Job drawing, mm, ordinate dimensions from the low corner. One solid piece. A direction names the side the tool comes from. Give positions to 0.01 mm unless a question says otherwise; leave off trailing zeros. Write each loop counter-clockwise with the first axis right and the second up, starting at its lowest first coordinate (ties: lowest second). Pieces come first, ordered by that corner, then holes. Notation, with made-up numbers: M -25,19.25 L 3,19.25 A24 ccw 3,30.25 Z; hole C 36.25,-38.5 d6. An arc over 180 degrees is marked long. Answer as CSV lines item,"result". Start each with the question number.
Item 1: Band-saw the part on C-C, the plane y = 2. List the corners of the cut face in (x, z) (1 decimal).
Item 2: Band-saw the part on A-A, the plane x = 31.3. List the corners of the cut face in (y, z).
Item 3: 3-axis set-ups, long thin cutter, end or side, ignore diameter. For the marked faces 4, 5, 6, 7 and 8: which of +Z, -Z, +X, -X, +Y, -Y reach the whole face in a straight line?
Item 4: Pin check, flat tips, straight feed: pin 1 (6 mm diameter, centred on y = 8.5, z = 21, fed in from +X); pin 2 (4 mm diameter, centred on x = 15.5, y = 8, fed in from -Z); pin 3 (1.5 mm diameter, centred on x = 31, y = 4.5, fed in from +Z); pin 4 (3 mm diameter, centred on x = 31.3, y = 6, fed in from +Z). Stop position of each tip, or through.
Item 5: Wall check: L1, parallel to Y at x = 31.3, z = 12; L2, parallel to Z at x = 29, y = 1; L3, parallel to Z at x = 14.5, y = 1.25. Give the ranges that are in metal, low to high. Write a range as from..to.
Item 6: Two-plate mould, pull along X, no slides. Class the marked faces 1, 2 and 3: +X half, -X half, draft (parallel to the pull), parting line (faces both ways), or undercut.
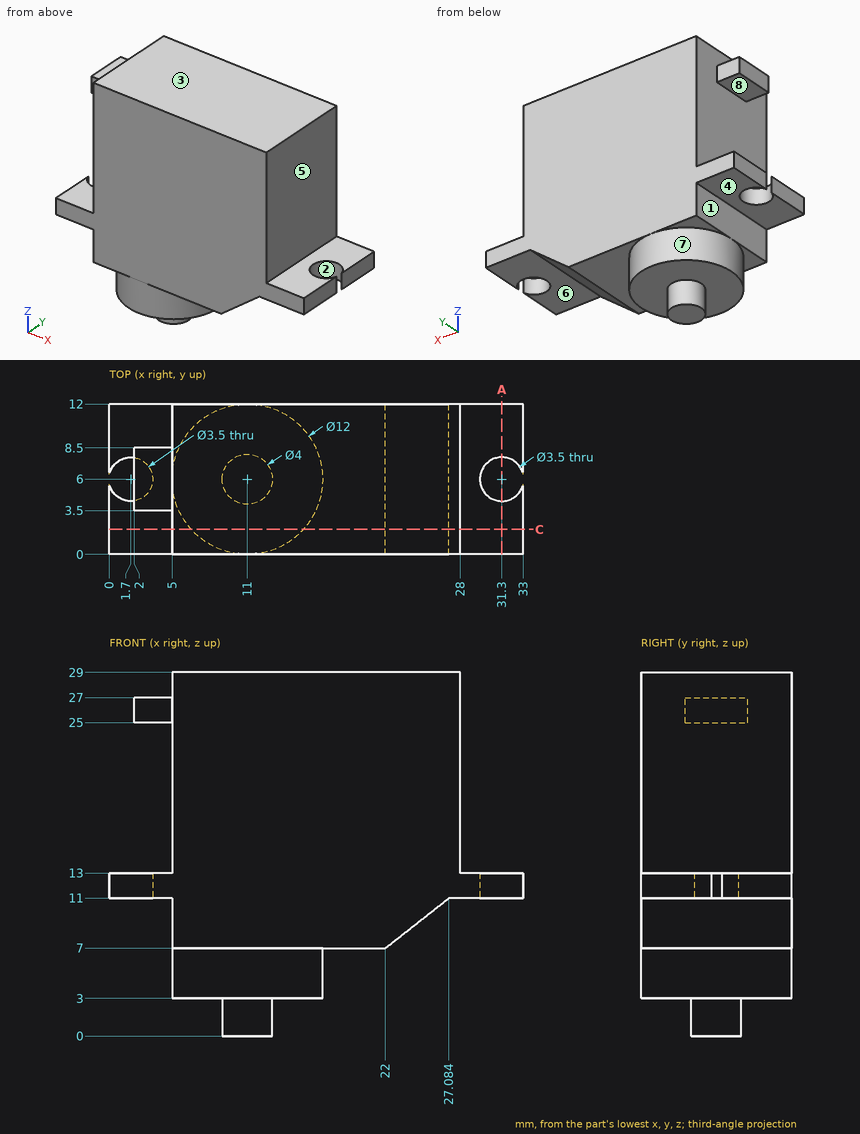
Output:
1,outline,"M 0,11 L 5,11 L 5,7 L 6.5,7 L 6.5,3 L 15.5,3 L 15.5,7 L 22,7 L 27.1,11 L 33,11 L 33,13 L 28,13 L 28,29 L 5,29 L 5,13 L 0,13 Z"
2,outline,"M 0,11 L 4.25,11 L 4.25,13 L 0,13 Z; M 7.75,11 L 12,11 L 12,13 L 7.75,13 Z"
3,face 4,"-Z, -X, +Y, -Y"
3,face 5,"+Z, +X, +Y, -Y"
3,face 6,"-Z, +X, +Y, -Y"
3,face 7,"-Z"
3,face 8,"-X, +Y, -Y"
4,pin 1,"x = 28"
4,pin 2,"z = 3"
4,pin 3,"z = 13"
4,pin 4,"through"
5,L1,"0..4.25, 7.75..12"
5,L2,"11..13"
5,L3,"3..29"
6,face 1,"-X half"
6,face 2,"undercut"
6,face 3,"draft"
